```python
from build123d import *

# Parameters (mm, degrees)
SKETCH1_W         = 38.1
SKETCH1_H         = 166
SKETCH1_R         = 11.509375
SKETCH1_R_2       = 3.571875
EXTRUSION1_DEPTH  = 25.4
EXTRUSION15_REACH = 171.009
SKETCH2_W         = 38.1
SKETCH2_H         = 9.170812283
EXTRUSION18_REACH = 90.865
SKETCH4_R         = 1.8
SKETCH4_W         = 5.953125
SKETCH4_H         = 166
SKETCH5_R         = 3.571875
SKETCH5_R_2       = 11.509375
EXTRUSION19_DEPTH = 5


with BuildPart() as part:
    # Sketch1 → Extrusion1 (new body)
    with BuildSketch(Plane(origin=(0, 0, 0), x_dir=(-1, 0, 0), z_dir=(0, 1, 0))):
        Rectangle(SKETCH1_W, SKETCH1_H)
        with Locations(Location((0, 0, 0), (0, 0, 270))):
            Circle(SKETCH1_R, mode=Mode.SUBTRACT)
        with Locations(Location((0, -44.45, 0), (0, 0, 270))):
            Circle(SKETCH1_R_2, mode=Mode.SUBTRACT)
        with Locations(Location((0, 44.45, 0), (0, 0, 270))):
            Circle(SKETCH1_R_2, mode=Mode.SUBTRACT)
    extrude(amount=EXTRUSION1_DEPTH)

    # Sketch2 → Extrusion15 (cut, up to next)
    with BuildSketch(Plane(origin=(0, 0, -83), x_dir=(-1, 0, 0), z_dir=(0, 0, -1)), mode=Mode.PRIVATE) as extrusion15_sk1:
        with Locations((0, 20.814593859)):
            Rectangle(SKETCH2_W, SKETCH2_H)
    extrusion15_tool1 = extrude(extrusion15_sk1.sketch, amount=-EXTRUSION15_REACH, mode=Mode.PRIVATE) & part.part
    add(extrusion15_tool1.solids().sort_by_distance((0, 20.814594, -83))[0], mode=Mode.SUBTRACT)

    # Sketch4 → Extrusion18 (cut, up to next)
    with BuildSketch(Plane(origin=(0, 25.4, 0), x_dir=(1, 0, 0), z_dir=(0, 1, 0)), mode=Mode.PRIVATE) as extrusion18_sk1:
        with Locations(Location((8.096875, -34, 0), (0, 0, 270))):
            Circle(SKETCH4_R)
    extrusion18_tool1 = extrude(extrusion18_sk1.sketch, amount=-EXTRUSION18_REACH, mode=Mode.PRIVATE) & part.part
    # Sketch4 → Extrusion18 (cut, up to next)
    with BuildSketch(Plane(origin=(0, 25.4, 0), x_dir=(1, 0, 0), z_dir=(0, 1, 0)), mode=Mode.PRIVATE) as extrusion18_sk2:
        with Locations(Location((8.096875, -27, 0), (0, 0, 270))):
            Circle(SKETCH4_R)
    extrusion18_tool2 = extrude(extrusion18_sk2.sketch, amount=-EXTRUSION18_REACH, mode=Mode.PRIVATE) & part.part
    # Sketch4 → Extrusion18 (cut, up to next)
    with BuildSketch(Plane(origin=(0, 25.4, 0), x_dir=(1, 0, 0), z_dir=(0, 1, 0)), mode=Mode.PRIVATE) as extrusion18_sk3:
        with Locations(Location((8.096875, -20, 0), (0, 0, 270))):
            Circle(SKETCH4_R)
    extrusion18_tool3 = extrude(extrusion18_sk3.sketch, amount=-EXTRUSION18_REACH, mode=Mode.PRIVATE) & part.part
    # Sketch4 → Extrusion18 (cut, up to next)
    with BuildSketch(Plane(origin=(0, 25.4, 0), x_dir=(1, 0, 0), z_dir=(0, 1, 0)), mode=Mode.PRIVATE) as extrusion18_sk4:
        with Locations(Location((8.096875, 20, 0), (0, 0, 270))):
            Circle(SKETCH4_R)
    extrusion18_tool4 = extrude(extrusion18_sk4.sketch, amount=-EXTRUSION18_REACH, mode=Mode.PRIVATE) & part.part
    # Sketch4 → Extrusion18 (cut, up to next)
    with BuildSketch(Plane(origin=(0, 25.4, 0), x_dir=(1, 0, 0), z_dir=(0, 1, 0)), mode=Mode.PRIVATE) as extrusion18_sk5:
        with Locations(Location((8.096875, 27, 0), (0, 0, 270))):
            Circle(SKETCH4_R)
    extrusion18_tool5 = extrude(extrusion18_sk5.sketch, amount=-EXTRUSION18_REACH, mode=Mode.PRIVATE) & part.part
    # Sketch4 → Extrusion18 (cut, up to next)
    with BuildSketch(Plane(origin=(0, 25.4, 0), x_dir=(1, 0, 0), z_dir=(0, 1, 0)), mode=Mode.PRIVATE) as extrusion18_sk6:
        with Locations(Location((8.096875, 34, 0), (0, 0, 270))):
            Circle(SKETCH4_R)
    extrusion18_tool6 = extrude(extrusion18_sk6.sketch, amount=-EXTRUSION18_REACH, mode=Mode.PRIVATE) & part.part
    # Sketch4 → Extrusion18 (cut, up to next)
    with BuildSketch(Plane(origin=(0, 25.4, 0), x_dir=(1, 0, 0), z_dir=(0, 1, 0)), mode=Mode.PRIVATE) as extrusion18_sk7:
        with Locations((-16.0734375, 0)):
            Rectangle(SKETCH4_W, SKETCH4_H)
    extrusion18_tool7 = extrude(extrusion18_sk7.sketch, amount=-EXTRUSION18_REACH, mode=Mode.PRIVATE) & part.part
    # Sketch4 → Extrusion18 (cut, up to next)
    with BuildSketch(Plane(origin=(0, 25.4, 0), x_dir=(1, 0, 0), z_dir=(0, 1, 0)), mode=Mode.PRIVATE) as extrusion18_sk8:
        with Locations((16.0734375, 0)):
            Rectangle(SKETCH4_W, SKETCH4_H)
    extrusion18_tool8 = extrude(extrusion18_sk8.sketch, amount=-EXTRUSION18_REACH, mode=Mode.PRIVATE) & part.part
    add(extrusion18_tool1.solids().sort_by_distance((8.096875, 25.4, 34))[0], mode=Mode.SUBTRACT)
    add(extrusion18_tool2.solids().sort_by_distance((8.096875, 25.4, 27))[0], mode=Mode.SUBTRACT)
    add(extrusion18_tool3.solids().sort_by_distance((8.096875, 25.4, 20))[0], mode=Mode.SUBTRACT)
    add(extrusion18_tool4.solids().sort_by_distance((8.096875, 25.4, -20))[0], mode=Mode.SUBTRACT)
    add(extrusion18_tool5.solids().sort_by_distance((8.096875, 25.4, -27))[0], mode=Mode.SUBTRACT)
    add(extrusion18_tool6.solids().sort_by_distance((8.096875, 25.4, -34))[0], mode=Mode.SUBTRACT)
    add(extrusion18_tool7.solids().sort_by_distance((-16.073437, 25.4, 0))[0], mode=Mode.SUBTRACT)
    add(extrusion18_tool8.solids().sort_by_distance((16.073438, 25.4, 0))[0], mode=Mode.SUBTRACT)

    # Sketch5 → Extrusion19 (add)
    with BuildSketch(Plane.XZ):
        with Locations(Location((0, 44.45, 0), (0, 0, 270))):
            Circle(SKETCH5_R)
        with Locations(Location((0, -44.45, 0), (0, 0, 270))):
            Circle(SKETCH5_R)
        with Locations(Location((0, 0, 0), (0, 0, 270))):
            Circle(SKETCH5_R_2)
    extrude(amount=-EXTRUSION19_DEPTH)


solid = part.part
```
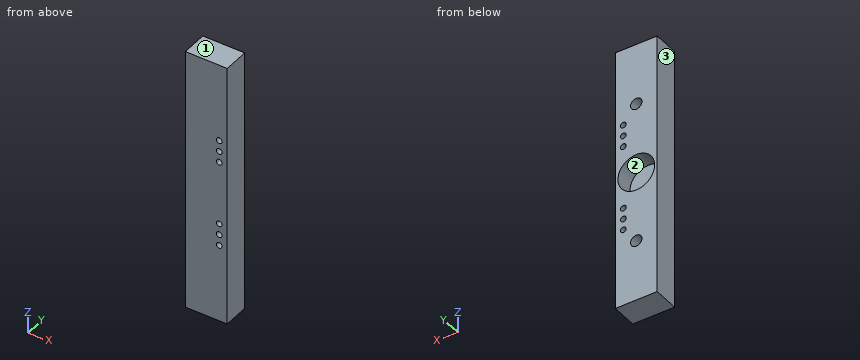
Read the model definition and answer for the solid it produces. Units are mm, in the model's axes. Face numbers are marked on the shaded views. Give positions to 0.01 mm unless a question says otherwise; leave off trailing zeros. Order: outer loops, then holes, each group sorted by start corner. A loop starts at its lowest first (then second) coordinate and runs counter-clockwise, first axis right, second up. Notation, with made-up numbers: (15, 52.25) -> (36, 52.25) arc R24 ccw to (36, 82.25) -> close; hole circle Ø9 at (13.5, 5). An arc over 180 degrees is marked (long way). One line per item, written item: value. Start each with the question number.
(1) The part is cut by section D-D (y = 7.75). State how many separate pieces and enclosed holes the cut face has, and give its area (3 significant figures).
(2) The part is cut by section A-A (z = -27). Determine the outline of the cut face in (x, y), and give its area (3 significant figures).
(3) The part is cut by section B-B (x = 0). Determine the outline of the cut face in (y, z).
(4) For a pull along X with two mould halves and no side action, classify the marked faces 1, 2 and 3 as released by +X, released by -X, zero draft, split by the parting line, or undercut.
(5) Straight lines are drawn through the part: L1, parallel to X at y = 11.25, z = 27; L2, parallel to Z at x = 0.5, y = 11.5; L3, parallel to Z at x = -1.5, y = 6.25. For each, find the intervals that lie inside material, in ascending order.
(6) Flat-ended cylindrical pins translate along their axes: P1, Ø2, axis at x = 2, z = -46, coming from the +Y side; P2, Ø3, axis at x = 8.1, z = 27, coming from the -Y side. Find the tip coordinate at first contact, or state that the pin passes through.
(7) The part is cut by section C-C (z = 44.45). Determine the outline of the cut face in (x, y), and give its area (3 significant figures).
Taken from the geometry:
1. separate pieces: 1
1. enclosed holes: 9
1. area: 3,790 mm^2
2. outline: (-13.1, 0) -> (6.3, 0) -> (6.3, 16.23) -> (-13.1, 16.23) -> close; (9.9, 0) -> (13.1, 0) -> (13.1, 16.23) -> (9.9, 16.23) -> close
2. area: 367 mm^2
3. outline: (0, -83) -> (16.23, -83) -> (16.23, -48.02) -> (5, -48.02) -> (5, -40.88) -> (16.23, -40.88) -> (16.23, -11.51) -> (5, -11.51) -> (5, 11.51) -> (16.23, 11.51) -> (16.23, 40.88) -> (5, 40.88) -> (5, 48.02) -> (16.23, 48.02) -> (16.23, 83) -> (0, 83) -> close
4. face 1: zero draft
4. face 2: undercut
4. face 3: released by -X
5. L1: -13.1 to 6.3, 9.9 to 13.1
5. L2: -83 to -47.99, -40.91 to -11.5, 11.5 to 40.91, 47.99 to 83
5. L3: -83 to -47.69, -41.21 to -11.41, 11.41 to 41.21, 47.69 to 83
6. P1: y = 5
6. P2: through
7. outline: (-13.1, 0) -> (13.1, 0) -> (13.1, 16.23) -> (3.57, 16.23) -> (3.57, 5) -> (-3.57, 5) -> (-3.57, 16.23) -> (-13.1, 16.23) -> close
7. area: 345 mm^2
